Geometry check sheet. Reference: the model listing, model coordinates, mm. Face numbers are marked on the shaded views. A direction names the side the tool comes from. Round coordinates to 2 decimals unless told otherwise and drop trailing zeros. Order: outer loops, then holes, each group sorted by start corner. A loop starts at its lowest first (then second) coordinate and runs counter-clockwise, first axis right, second up. Notation, with made-up numbers: (1.25, 68) - (42.25, 68) arc R7 cw to (42.25, 79) - close; hole circle Ø5 at (-5.5, 71). An arc over 180 degrees is marked (long way). Write each question's results on one line, items separated by ' | '.
```python
from build123d import *

# Parameters (mm, degrees)
F1_DEPTH  = 28.575
F3_DEPTH  = 31.75
F5_DEPTH  = 69.851
F6_R      = 6.35
F7_DEPTH  = 25.401
F9_DEPTH  = 25.401
F11_DEPTH = 25.401


with BuildPart() as f1:
    # F0 (on Front) → F1 (new body, symmetric)
    with BuildSketch(Plane.XZ):
        Polygon((0, 6.35), (0, 0), (101.6, 0), (101.6, 31.75), (44.45, 69.85), (-6.35, 69.85), (-6.35, 6.35), align=None)
    extrude(amount=F1_DEPTH, both=True)

    # F2 (on face) → F3 (cut)
    with BuildSketch(Plane.XZ.offset(28.575)):
        Polygon((38.1, 0), (101.6, 0), (101.6, 31.75), (44.45, 69.85), (-6.35, 69.85), (-6.35, 31.75), (38.1, 31.75), (38.1, 19.05), (50.8, 19.05), (50.8, 12.7), (38.1, 12.7), align=None)
    extrude(amount=-F3_DEPTH, mode=Mode.SUBTRACT)

    # F4 (on face) → F5 (cut, through all)
    with BuildSketch(Plane(origin=(0, 0, 0), x_dir=(1, 0, 0), z_dir=(0, 0, -1))):
        Polygon((85.725, -28.575), (101.6, -28.575), (101.6, -12.7), align=None)
    extrude(amount=-F5_DEPTH, mode=Mode.SUBTRACT)

    # F6 (on face) → F7 (cut, through all)
    with BuildSketch(Plane.XZ.offset(-3.175)):
        with Locations((12.699999, 50.8)):
            Circle(F6_R)
    extrude(amount=-F7_DEPTH, mode=Mode.SUBTRACT)

    # F8 (on face) → F9 (cut, through all)
    with BuildSketch(Plane.XZ.offset(-3.175)):
        Polygon((38.1, 12.7), (38.1, 0), (101.6, 0), (101.6, 12.7), (50.8, 12.7), align=None)
    extrude(amount=-F9_DEPTH, mode=Mode.SUBTRACT)

    # F10 (on face) → F11 (cut, through all)
    with BuildSketch(Plane.XZ.offset(-3.175)):
        Polygon((44.45, 69.85), (-6.35, 69.85), (-6.35, 63.5), (53.975, 63.5), align=None)
    extrude(amount=-F11_DEPTH, mode=Mode.SUBTRACT)


solid = f1.part
```
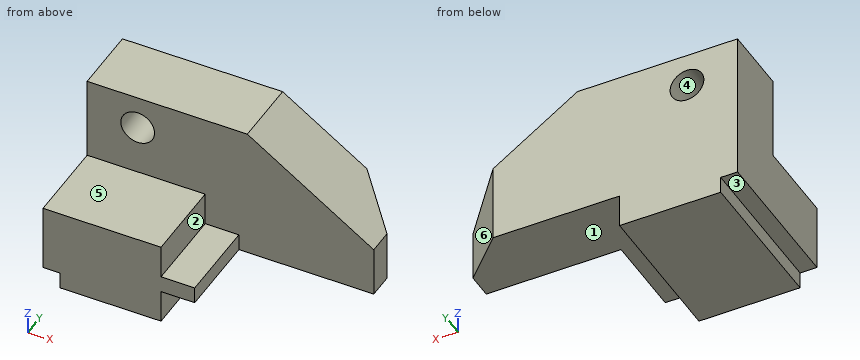
(1) Section check C-C (y = -16.5). Record the cut outline in (x, z), then the cut area to 3 significant figures.
Answers follow:
outline: (-6.35, 6.35) - (0, 6.35) - (0, 0) - (38.1, 0) - (38.1, 12.7) - (50.8, 12.7) - (50.8, 19.05) - (38.1, 19.05) - (38.1, 31.75) - (-6.35, 31.75) - close | area: 1,450 mm²
(2) Material ranges on line 1 (Z direction, x = 12.7, y = 21); line 2 (Z direction, x = 8, y = -22); line 3 (Y direction, x = 17, z = 56) (3 decimals), recorded low to high.
Answers follow:
line 1: 0 to 44.45, 57.15 to 63.5 | line 2: 0 to 31.75 | line 3: 3.175 to 28.575
(3) Depth check by flat-ended pin: pin 1 Ø7 at (y, z) = (-11.5, 16.5) entering from +X; pin 2 Ø2 at (x, y) = (55.5, 0.5) entering from +Z; pin 3 Ø5 at (x, y) = (45.5, 9) entering from -Z; pin 4 Ø4 at (y, z) = (-15, 23.5) entering from +X. Enter the tip coordinate at first touch or a pass-through.
Answers follow:
pin 1: x = 50.8 | pin 2: through | pin 3: z = 12.7 | pin 4: x = 38.1
(4) Section check D-D (z = 30). Record the cut outline in (x, y) (3 decimals), then the cut area to 3 significant figures.
Answers follow:
outline: (-6.35, -28.575) - (38.1, -28.575) - (38.1, 3.175) - (101.6, 3.175) - (101.6, 12.7) - (85.725, 28.575) - (-6.35, 28.575) - close | area: 4,030 mm²
(5) Section check A-A (x = 12.7). Record the cut outline in (y, z) (3 decimals).
Answers follow:
outline: (-28.575, 0) - (28.575, 0) - (28.575, 44.45) - (3.175, 44.45) - (3.175, 31.75) - (-28.575, 31.75) - close; (3.175, 57.15) - (28.575, 57.15) - (28.575, 63.5) - (3.175, 63.5) - close
(6) Access from +Z, -Z, +X, -X, +Y, -Y to the whole of each face (thin tool, end or side, straight path). Record for the marked faces 1, 2 and 3.
Answers follow:
face 1: -Z, +X, +Y, -Y | face 2: +Z, +X, -Y | face 3: -Z, -X, +Y, -Y
(7) Section check B-B (z = 56). Record the cut outline in (x, y) (3 decimals), then the cut area to 3 significant figures.
Answers follow:
outline: (-6.35, 3.175) - (9.055, 3.175) - (9.055, 28.575) - (-6.35, 28.575) - close; (16.345, 3.175) - (65.225, 3.175) - (65.225, 28.575) - (16.345, 28.575) - close | area: 1,630 mm²
(8) Draft check along X on the marked faces 4, 5 and 6. Enter one of: released by +X, released by -X, zero draft, split by the parting line, or undercut.
Answers follow:
face 4: undercut | face 5: zero draft | face 6: released by +X
